```python
from build123d import *

# Parameters (mm, degrees)
F0_R     = 6
F1_DEPTH = 2
F2_SIZE2 = 2.5980762114
F2_SIZE  = 1.5
F4_R     = 2.85
F4_R_2   = 1.4
F5_DEPTH = 4.5
F6_R     = 1.2


# Not quite as in the source:
# - a fillet or chamfer that OpenCascade refuses, or shapes differently, is made with other operations: its cross-section is extruded or revolved along the edge and cut away or added


with BuildPart() as f1:
    # F0 (on Top) → F1 (new body)
    with BuildSketch(Plane.XY):
        Circle(F0_R)
    extrude(amount=F1_DEPTH)

    # F2
    f2_edges = [f1.edges().sort_by_distance(p)[0] for p in [
        (-6, 0, 0),
    ]]
    f2_side = f1.faces().sort_by_distance((-6, 0, 1))[0]
    chamfer(f2_edges, length=F2_SIZE, length2=F2_SIZE2, reference=f2_side)

    # F3: fillet of radius 1 on 2 edges, made by hand

    # F3_s1 → F3_t2 (revolve, cut)
    with BuildSketch(Plane.XZ):
        with BuildLine():
            ThreePointArc((3.6339745962, 0.1339745962), (3.3927936413, 0.0340741737), (3.1339745962, 0))
            Line((3.1339745962, 0), (3.4019237886, 0))
            Line((3.4019237886, 0), (3.6339745962, 0.1339745962))
        make_face()
    revolve(axis=Axis((0, 0, 0), (0, 0, 1)), mode=Mode.SUBTRACT)

    # F3_s3 → F3_t4 (revolve, cut)
    with BuildSketch(Plane.XZ):
        with BuildLine():
            ThreePointArc((6, 2), (5.8486778537, 1.5452494356), (5.5031382462, 1.2131367327))
            Line((5.5031382462, 1.2131367327), (6, 1.5))
            Line((6, 1.5), (6, 2))
        make_face()
    revolve(axis=Axis((0, 0, 1.5), (0, 0, 1)), mode=Mode.SUBTRACT)

    # F4 (on face) → F5 (join)
    with BuildSketch(Plane.XY.offset(2)):
        Circle(F4_R)
        Circle(F4_R_2, mode=Mode.SUBTRACT)
    extrude(amount=F5_DEPTH)

    # F6
    f6_edges = [f1.edges().sort_by_distance(p)[0] for p in [
        (-1.4, 0, 2),
    ]]
    fillet(f6_edges, radius=F6_R)


solid = f1.part
```
Here's how the part is built. I have some questions about the finished solid (model axes, mm). Give positions to 0.01 mm unless a question says otherwise; leave off trailing zeros. Order: outer loops, then holes, each group sorted by start corner. A loop starts at its lowest first (then second) coordinate and runs counter-clockwise, first axis right, second up. Notation, with made-up numbers: (29.5, -20) - (37.5, -20) arc R20 ccw to (37.5, -2) - close; hole circle Ø8 at (23, -32). An arc over 180 degrees is marked (long way). Answer as a JSON object with one key per item and string values. Group by question number.
Item 1: If we section it at A-A on z = 3.75: Please give me the cut outline in (x, y), and give its area (3 significant figures).
Item 2: If we mould it in two halves opening along X, with no side actions, what happens to faces 1 (the cylindrical face through (-2.262, -1.734, 4.219)), 2 (the cylindrical face through (-1.4, 0.06, 4.83)), 3 (the flat face through (3, -1, 2))? For each: pulls with the +X half, pulls with the -X half, needs draft (parallel to the pull), parting line crosses it, or undercut.
Item 3: Please list where these lines run through material, in increasing order: probe 1 along Y at (x, z) = (0, 5); probe 2 along X at (y, z) = (2.5, 0.5); probe 3 along Z at (x, y) = (-1.25, 3.5).
Item 4: For P1, Ø2, axis at y = -2.5, z = 3.5, coming from the +X side, with a flat end and sliding along its axis, tell me the tip position at first contact or that it passes through.
Result set:
{
 "1": {"outline": "circle Ø5.7 at (0, 0); hole circle Ø2.8 at (0, 0)", "area": "19.4 mm²"},
 "2": {"face 1": "parting line crosses it", "face 2": "undercut", "face 3": "needs draft"},
 "3": {"probe 1": "-2.85 to -1.4, 1.4 to 2.85", "probe 2": "-3.46 to 3.46", "probe 3": "0.18 to 2"},
 "4": {"P1": "x = 2.42"}
}
